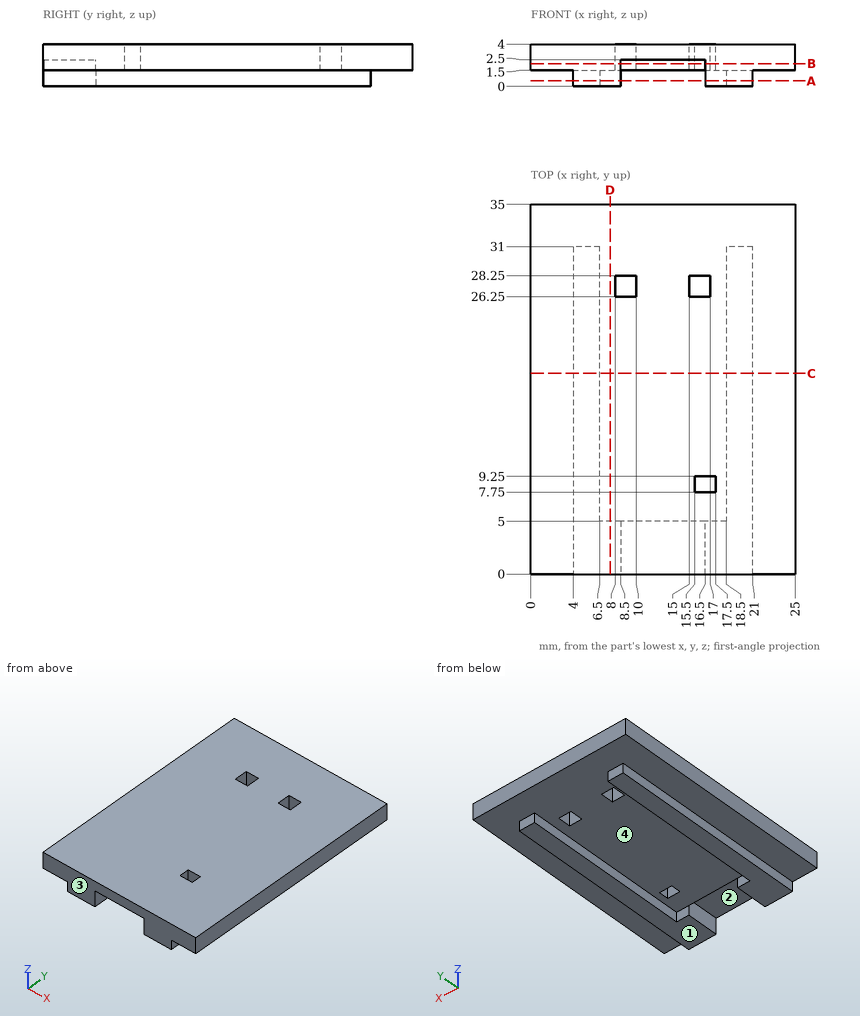
For this review, use the dimensioned drawing (mm, ordinates from the lowest corner) and the shaded views. A direction names the side the tool comes from. Round coordinates to 2 decimals unless told otherwise and drop trailing zeros. Write each loop counter-clockwise with the first axis right and the second up, starting at its lowest first coordinate (ties: lowest second). Pieces come first, ordered by that corner, then holes. Notation, with made-up numbers: (-27, 79) -> (-14, 79) arc R32 ccw to (-14, 114) -> close; hole circle Ø11 at (-10.5, 33). An arc over 180 degrees is marked (long way). Use one line per item in the form item = value.
Q1. The part is to be moulded in two halves that separate along X. For the marked faces 3 and 4, say which applies: released by +X, released by -X, zero draft, split by the parting line, or undercut.
Resolved:
face_3 = zero draft
face_4 = undercut
Q2. Consider section B-B (z = 2.15). State the section outline as (x, y) points.
Resolved:
outline = (0, 0) -> (8.5, 0) -> (8.5, 5) -> (16.5, 5) -> (16.5, 0) -> (25, 0) -> (25, 35) -> (0, 35) -> close; hole (8, 26.25) -> (10, 26.25) -> (10, 28.25) -> (8, 28.25) -> close; hole (15, 26.25) -> (17, 26.25) -> (17, 28.25) -> (15, 28.25) -> close; hole (15.5, 7.75) -> (17.5, 7.75) -> (17.5, 9.25) -> (15.5, 9.25) -> close
Q3. To check wall thickness, follow probe 1 along X at (y, z) = (22, 1.2); probe 2 along Y at (x, z) = (20, 0.4); probe 3 along X at (y, z) = (8.5, 2.1). State the ranges of each line that lie inside material, in increasing order. Write a range as from..to.
Resolved:
probe_1 = 4..6.5, 18.5..21
probe_2 = 0..31
probe_3 = 0..15.5, 17.5..25
Q4. Consider section D-D (x = 7.5). State the section outline as (y, z) points.
Resolved:
outline = (0, 0) -> (5, 0) -> (5, 1.5) -> (35, 1.5) -> (35, 4) -> (0, 4) -> close
Q5. Clearance check with flat-ended pins moving along their axes: pin 1 Ø1.6 at (y, z) = (19.5, 0.5) entering from -X; pin 2 Ø1.6 at (y, z) = (18, 0.5) entering from +X. State where each tip first meets the part, or that it passes through.
Resolved:
pin_1 = 4
pin_2 = 21
Q6. Consider section C-C (y = 19). State the section outline as (x, z) points.
Resolved:
outline = (0, 1.5) -> (4, 1.5) -> (4, 0) -> (6.5, 0) -> (6.5, 1.5) -> (18.5, 1.5) -> (18.5, 0) -> (21, 0) -> (21, 1.5) -> (25, 1.5) -> (25, 4) -> (0, 4) -> close
Q7. Machinability: for the marked faces 1 and 2, which of the approach directions +Z, -Z, +X, -X, +Y, -Y give a long, thin tool a straight path to every point of the face, cutting with its end or side? Answer none if there is none.
Resolved:
face_1 = -Z, +X, -X, +Y, -Y
face_2 = -Z, -Y
Q8. Consider section A-A (z = 0.5). State the section outline as (x, y) points.
Resolved:
outline = (4, 0) -> (8.5, 0) -> (8.5, 5) -> (6.5, 5) -> (6.5, 31) -> (4, 31) -> close; (16.5, 0) -> (21, 0) -> (21, 31) -> (18.5, 31) -> (18.5, 5) -> (16.5, 5) -> close
